Read the model definition and answer for the solid it produces. Units are mm, in the model's axes. A direction names the side the tool comes from. Coordinates: 2 decimals unless noted, no trailing zeros. Order: outer loops, then holes, each group sorted by start corner. A loop starts at its lowest first (then second) coordinate and runs counter-clockwise, first axis right, second up.
from build123d import *
from build123d.topology import SkipClean

# Parameters (mm, degrees)
BOSS_EXTRU_1_DEPTH      = 5
BOSS_EXTRU_3_START      = 2
BOSS_EXTRU_3_DEPTH      = 2
ESQUISSE5_R             = 0.5
ESQUISSE5_R_2           = 2.5
ENL_V_MAT_EXTRU_1_DEPTH = 2
ESQUISSE7_R             = 2.5
ENL_V_MAT_EXTRU_2_DEPTH = 24.906066176
ESQUISSE8_R             = 2
ENL_V_MAT_EXTRU_3_DEPTH = 26.719642463


with BuildPart() as part:
    # Esquisse1 → Boss.-Extru.1 (new body)
    with BuildSketch(Plane.XY):
        with BuildLine():
            Line((-1.732050808, 1), (1.732050808, 1))
            ThreePointArc((1.732050808, 1), (1.931851653, 0.51763809), (2, 0))
            Line((2, 0), (17.5, 0))
            ThreePointArc((17.5, 0), (0, 17.5), (-17.5, 0))
            Line((-17.5, 0), (-2, 0))
            ThreePointArc((-2, 0), (-1.931851653, 0.51763809), (-1.732050808, 1))
        make_face()
    extrude(amount=BOSS_EXTRU_1_DEPTH)

    # Esquisse3 → Boss.-Extru.3 (add)
    with SkipClean():  # the faces are left unmerged after this step: merging them gives an invalid solid
        with BuildSketch(Plane(origin=(0, 0, 0), x_dir=(-1, 0, 0), z_dir=(0, 0, -1)).offset(BOSS_EXTRU_3_START)):
            with BuildLine():
                Line((0, 2), (0, 17.5))
                ThreePointArc((0, 17.5), (-12.374368671, 12.374368671), (-17.5, 0))
                Line((-17.5, 0), (-2, 0))
                ThreePointArc((-2, 0), (-1.931851653, 0.51763809), (-1.732050808, 1))
                ThreePointArc((-1.732050808, 1), (-1, 1.732050808), (0, 2))
            make_face()
            with BuildLine():
                ThreePointArc((17.5, 0), (12.374368671, 12.374368671), (0, 17.5))
                Line((0, 17.5), (0, 2))
                ThreePointArc((0, 2), (1, 1.732050808), (1.732050808, 1))
                ThreePointArc((1.732050808, 1), (1.931851653, 0.51763809), (2, 0))
                Line((2, 0), (17.5, 0))
            make_face()
        extrude(amount=-BOSS_EXTRU_3_DEPTH)

    # Esquisse5 → Enlèv. mat.-Extru.1 (cut)
    with SkipClean():  # the faces are left unmerged after this step: merging them gives an invalid solid
        with BuildSketch(Plane.XZ):
            with Locations(Location((-10.5, 1.5, 0), (0, 0, 270))):
                Circle(ESQUISSE5_R)
            with Locations(Location((10.5, 1.5, 0), (0, 0, 270))):
                Circle(ESQUISSE5_R_2)
        extrude(amount=-ENL_V_MAT_EXTRU_1_DEPTH, mode=Mode.SUBTRACT)

    # Esquisse7 → Enlèv. mat.-Extru.2 (cut, through all)
    with SkipClean():  # the faces are left unmerged after this step: merging them gives an invalid solid
        with BuildSketch(Plane.XZ.offset(-2)):
            with Locations(Location((10.5, 1.5, 0), (0, 0, 270))):
                Circle(ESQUISSE7_R)
        extrude(amount=-ENL_V_MAT_EXTRU_2_DEPTH, mode=Mode.SUBTRACT)

    # Esquisse8 → Enlèv. mat.-Extru.3 (cut, through all)
    with SkipClean():  # the faces are left unmerged after this step: merging them gives an invalid solid
        with BuildSketch(Plane(origin=(0, 0, -2), x_dir=(-1, 0, 0), z_dir=(0, 0, -1))):
            Circle(ESQUISSE8_R)
        extrude(amount=-ENL_V_MAT_EXTRU_3_DEPTH, mode=Mode.SUBTRACT)


solid = part.part
Q1. Which of the six approach directions +Z, -Z, +X, -X, +Y, -Y give full straight-line access (tool end or side, diameter ignored) to faces 1 (the cylindrical face through (-10.988, 0.986, 1.608)), 2 (the flat face through (-10, 0, 1))?
Q2. The part is cut by section C-C, the plane x = -10.5. Determine the outline of the cut face in (y, z), then the cut area to 3 significant figures.
Q3. The part is cut by section A-A, the plane x = 10.5. Determine the outline of the cut face in (y, z).
Q4. Straight lines are drawn through the part: L1, parallel to X at y = 1.5, z = 0; L2, parallel to X at y = 1.55, z = 1.5; L3, parallel to Z at x = 10.5, y = 9. For each, find the intervals that lie inside material, in ascending order.
Q5. The part is cut by section B-B, the plane z = 2.75. Determine the outline of the cut face in (x, y).
Q6. Determine the mould class of faces 3 (the flat face through (-10.5, 2, 1.5)), 4 (the cylindrical face through (0, 2, 1)), 5 (the flat face through (0, 7, -2)) for opening direction Z: +Z half, -Z half, draft (parallel to the pull), parting line (faces both ways), or undercut.
Q7. The part is cut by section D-D, the plane y = 10. Determine the outline of the cut face in (x, z), then the cut area to 3 significant figures.
Computed values:
1. face 1: -Y
1. face 2: +Z, -Z, +X, -X, -Y
2. outline: (0, -2) - (14, -2) - (14, 5) - (0, 5) - (0, 2) - (2, 2) - (2, 1) - (0, 1) - close
2. area: 96.0 mm2
3. outline: (0, -2) - (14, -2) - (14, -1) - (0, -1) - close; (0, 4) - (14, 4) - (14, 5) - (0, 5) - close
4. L1: x = -17.44 to -1.32, 1.32 to 8.5, 12.5 to 17.44
4. L2: x = -17.43 to -11, -10 to -1.26, 1.26 to 8, 13 to 17.43
4. L3: z = -2 to -1, 4 to 5
5. outline: (-17.5, 0) - (-2, 0) arc R2 cw to (2, 0) - (8.33, 0) - (8.33, 15.39) arc R17.5 ccw to start; (12.67, 0) - (17.5, 0) arc R17.5 ccw to (12.67, 12.08) - close
6. face 3: undercut
6. face 4: draft
6. face 5: -Z half
7. outline: (-14.36, -2) - (14.36, -2) - (14.36, 5) - (-14.36, 5) - close; hole circle Ø5 at (10.5, 1.5)
7. area: 181 mm2
